from build123d import *

# Parameters (mm, degrees)
SKETCH1_W          = 140
SKETCH1_H          = 350
EXTRUDE1_DEPTH     = 20
CUT_EXTRUDE2_DEPTH = 10
SKETCH4_R          = 2.25
CUT_EXTRUDE3_DEPTH = 15
SKETCH6_R          = 2.25
CUT_EXTRUDE5_DEPTH = 15
SKETCH7_R          = 1.65
CUT_EXTRUDE6_DEPTH = 20


with BuildPart() as part:
    # Sketch1 → Extrude1 (new body)
    with BuildSketch(Plane.XY):
        with Locations((70, 175)):
            Rectangle(SKETCH1_W, SKETCH1_H)
    extrude(amount=EXTRUDE1_DEPTH)

    # Sketch3 → Cut-Extrude2 (cut)
    with BuildSketch(Plane(origin=(0, 0, 0), x_dir=(-1, 0, 0), z_dir=(0, 0, -1))):
        Polygon((-70, 350), (-55, 350), (-40, 350), (-40, 0), (-100, 0), (-100, 350), align=None)
    extrude(amount=-CUT_EXTRUDE2_DEPTH, mode=Mode.SUBTRACT)

    # Sketch4 → Cut-Extrude3 (cut)
    with BuildSketch(Plane(origin=(0, 350, 0), x_dir=(-1, 0, 0), z_dir=(0, 1, 0))):
        with Locations((-20, 10)):
            Circle(SKETCH4_R)
        with Locations((-70, 15)):
            Circle(SKETCH4_R)
        with Locations((-120, 10)):
            Circle(SKETCH4_R)
    extrude(amount=-CUT_EXTRUDE3_DEPTH, mode=Mode.SUBTRACT)

    # Sketch6 → Cut-Extrude5 (cut)
    with BuildSketch(Plane.XZ):
        with Locations((20, 10)):
            Circle(SKETCH6_R)
        with Locations((120, 10)):
            Circle(SKETCH6_R)
    extrude(amount=-CUT_EXTRUDE5_DEPTH, mode=Mode.SUBTRACT)

    # Sketch7 → Cut-Extrude6 (cut)
    with BuildSketch(Plane(origin=(0, 0, 0), x_dir=(-1, 0, 0), z_dir=(0, 0, -1))):
        with Locations((-123, 331)):
            Circle(SKETCH7_R)
        with Locations((-17, 331)):
            Circle(SKETCH7_R)
        with Locations((-17, 31)):
            Circle(SKETCH7_R)
        with Locations((-123, 31)):
            Circle(SKETCH7_R)
        with Locations((-17, 271)):
            Circle(SKETCH7_R)
        with Locations((-17, 211)):
            Circle(SKETCH7_R)
        with Locations((-17, 151)):
            Circle(SKETCH7_R)
        with Locations((-17, 91)):
            Circle(SKETCH7_R)
        with Locations((-123, 91)):
            Circle(SKETCH7_R)
        with Locations((-123, 151)):
            Circle(SKETCH7_R)
        with Locations((-123, 211)):
            Circle(SKETCH7_R)
        with Locations((-123, 271)):
            Circle(SKETCH7_R)
    extrude(amount=-CUT_EXTRUDE6_DEPTH, mode=Mode.SUBTRACT)


solid = part.part
Verification items for the finished model (mm, model axes). A direction names the side the tool comes from. Coordinates: 2 decimals unless noted, no trailing zeros. Order: outer loops, then holes, each group sorted by start corner. A loop starts at its lowest first (then second) coordinate and runs counter-clockwise, first axis right, second up.
1. Release check for a two-part mould opening along X. For faces 3 (the face through (100, 173, 5)), 4 (the face through (70, 177, 10)), 5 (the face through (69, 0, 12)), 6 (the face through (0, 173, 10)) record: +X half, -X half, draft (parallel to the pull), parting line (faces both ways), or undercut.
Results found:
face 3: undercut
face 4: undercut
face 5: draft
face 6: -X half
2. Sectioned sample at B-B, the plane y = 143.5. Record the cut outline in (x, z).
Results found:
outline: (0, 0) - (40, 0) - (40, 10) - (100, 10) - (100, 0) - (140, 0) - (140, 20) - (0, 20) - close
3. Scan lines: line 1 (X direction, y = 91, z = 11); line 2 (X direction, y = 151, z = 5); line 3 (X direction, y = 71.5, z = 5.5). Record each from-to range of solid material in increasing order.
Results found:
line 1: x = 0 to 15.35, 18.65 to 121.35, 124.65 to 140
line 2: x = 0 to 15.35, 18.65 to 40, 100 to 121.35, 124.65 to 140
line 3: x = 0 to 40, 100 to 140
4. Sectioned sample at C-C, the plane x = 76. Record the cut outline in (y, z).
Results found:
outline: (0, 10) - (350, 10) - (350, 20) - (0, 20) - close
5. Sectioned sample at A-A, the plane z = 3. Give the number of separate pieces and of enclosed holes in the cut face, and give its area (3 significant figures).
Results found:
separate pieces: 2
enclosed holes: 12
area: 27,900 mm2
6. Set-up check for faces 1 (the face through (20, 177, 0)), 2 (the face through (40, 177, 5)): record each of +Z, -Z, +X, -X, +Y, -Y from which the full face is reachable in a straight line by a thin tool's end or side.
Results found:
face 1: -Z, +X, -X, +Y, -Y
face 2: -Z, +Y, -Y
7. Go/stop test with flat-tipped pins: pin 1 Ø3 at (x, y) = (123, 331) entering from -Z; pin 2 Ø1.3 at (x, z) = (120.5, 11) entering from +Y; pin 3 Ø18 at (x, y) = (76, 94.5) entering from -Z; pin 4 Ø1.3 at (x, z) = (20, 10) entering from -Y. Record where each tip stops, or that it passes through.
Results found:
pin 1: passes through
pin 2: stops at y = 335
pin 3: stops at z = 10
pin 4: stops at y = 15
